Answer from the drawing. Dimensions are ordinates in mm from the lowest x, y and z of the part. A direction names the side the tool comes from. Coordinates: 2 decimals unless noted, no trailing zeros. Write each loop counter-clockwise with the first axis right and the second up, starting at its lowest first coordinate (ties: lowest second). Pieces come first, ordered by that corner, then holes.
1) The part is cut by section B-B (x = 12.5). Determine the outline of the cut face in (y, z), then the cut area to 3 significant figures.
2) The part is cut by section A-A (z = 1.2). Determine the outline of the cut face in (x, y), then the cut area to 3 significant figures.
3) Determine the mould class of the marked faces 1, 2, 3 and 4 for opening direction Y: +Y half, -Y half, draft (parallel to the pull), parting line (faces both ways), or undercut.
4) This flat-tipped pin is pushed along its axis until it touches: pin 1 Ø1 at (x, z) = (7.5, 2.5) entering from -Y. Where does it stop, or does it pass through?
5) Find the intervals of material crossed by line 1 (X direction, y = 1.5, z = 3.15); line 2 (Y direction, x = 12.5, z = 1.25); line 3 (X direction, y = 1.5, z = 1.4), in increasing order.
6) Which of the six approach directions +Z, -Z, +X, -X, +Y, -Y give full straight-line access (tool end or side, diameter ignored) to the marked faces 5, 6 and 7?
7) The part is cut by section C-C (y = 2.05). Determine the outline of the cut face in (x, z).
8) The part is cut by section D-D (z = 2.7). Determine the outline of the cut face in (x, y), then the cut area to 3 significant figures.
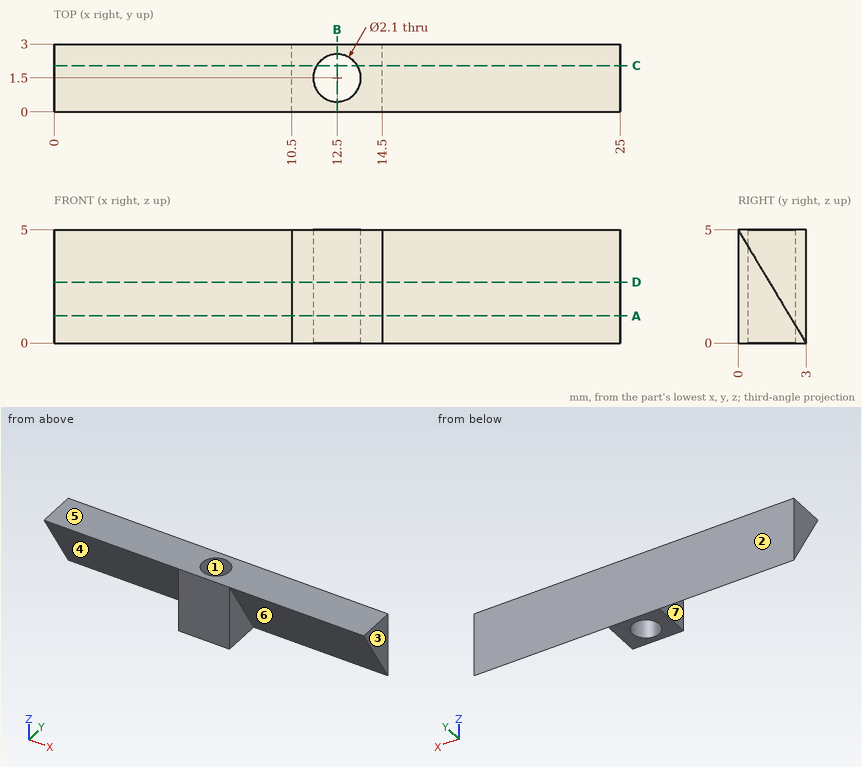
Reported:
1. outline: (0, 0) - (0.45, 0) - (0.45, 5) - (0, 5) - close; (2.55, 0) - (3, 0) - (3, 5) - (2.55, 5) - close
1. area: 4.50 mm2
2. outline: (0, 2.28) - (10.5, 2.28) - (10.5, 0) - (14.5, 0) - (14.5, 2.28) - (25, 2.28) - (25, 3) - (0, 3) - close; hole circle Ø2.1 at (12.5, 1.5)
2. area: 23.7 mm2
3. face 1: undercut
3. face 2: +Y half
3. face 3: draft
3. face 4: -Y half
4. pin 1: stops at y = 1.2
5. line 1: x = 0 to 11.45, 13.55 to 25
5. line 2: y = 0 to 0.45, 2.55 to 3
5. line 3: x = 10.5 to 11.45, 13.55 to 14.5
6. face 5: +Z, +X, -X, +Y, -Y
6. face 6: -Z, +X, -Y
6. face 7: -Z, -X, -Y
7. outline: (0, 1.58) - (10.5, 1.58) - (10.5, 0) - (11.61, 0) - (11.61, 5) - (0, 5) - close; (13.39, 0) - (14.5, 0) - (14.5, 1.58) - (25, 1.58) - (25, 5) - (13.39, 5) - close
8. outline: (0, 1.38) - (10.5, 1.38) - (10.5, 0) - (14.5, 0) - (14.5, 1.38) - (25, 1.38) - (25, 3) - (0, 3) - close; hole circle Ø2.1 at (12.5, 1.5)
8. area: 42.6 mm2
